```python
from build123d import *

# Parameters (mm, degrees)
F2_R     = 1
F3_SIZE  = 1
F5_DEPTH = 2.88


# Not quite as in the source:
# - a fillet or chamfer that OpenCascade refuses, or shapes differently, is made with other operations: its cross-section is extruded or revolved along the edge and cut away or added


with BuildPart() as f1:
    # F0 (on Front) → F1 (revolve)
    with BuildSketch(Plane.XZ):
        Polygon((-4, 0), (0, 0), (0, 51.056624327), (-2.5, 52.5), (-2.5, 58), (-6.5, 58), (-6.5, 50), (-4, 50), (-4, 46.25), (-3.5, 46), (-4, 45.75), align=None)
    revolve(axis=Axis((0, 0, 18.332445994), (0, 0, 1)))

    # F2
    f2_edges = [f1.edges().sort_by_distance(p)[0] for p in [
        (6.5, 0, 58),
    ]]
    fillet(f2_edges, radius=F2_R)

    # F3
    f3_edges = [f1.edges().sort_by_distance(p)[0] for p in [
        (4, 0, 0),
    ]]
    chamfer(f3_edges, length=F3_SIZE)

    # F4 (on face) → F5 (cut)
    with BuildSketch(Plane.XY.offset(58)):
        Polygon((-1.7320508076, -3), (1.7320508076, -3), (3.4641016151, 0), (1.7320508076, 3), (-1.7320508076, 3), (-3.4641016151, 0), align=None)
    extrude(amount=-F5_DEPTH, mode=Mode.SUBTRACT)

    # F6: chamfer of 1.5 x 2.5980762114 on 1 edges, made by hand


with BuildPart() as f6_tool2:
    # F6_s3 → F6_t4 (revolve)
    with BuildSketch(Plane.XZ):
        Polygon((-5.0980762114, 55.12), (-2.5, 53.62), (-2.5, 55.12), align=None)
    revolve(axis=Axis((0, 0, 55.12), (0, 0, 1)))

    split(bisect_by=Plane(origin=(-2.5980762114, -1.5, 0), x_dir=(0, 0, 1), z_dir=(0.8660254038, 0.5, 0)), keep=Keep.TOP)

    split(bisect_by=Plane(origin=(-2.5980762114, 1.5, 0), x_dir=(0, 0, 1), z_dir=(0.8660254038, -0.5, 0)), keep=Keep.TOP)

    split(bisect_by=Plane.XZ.offset(-3), keep=Keep.TOP)

    split(bisect_by=Plane(origin=(2.5980762114, 1.5, 0), x_dir=(0, 0, 1), z_dir=(-0.8660254038, -0.5, 0)), keep=Keep.TOP)

    split(bisect_by=Plane(origin=(2.5980762114, -1.5, 0), x_dir=(0, 0, 1), z_dir=(-0.8660254038, 0.5, 0)), keep=Keep.TOP)

    split(bisect_by=Plane.XZ.offset(3), keep=Keep.BOTTOM)


with BuildPart() as f1_1:
    add(f1.part)

    # F6_t1: cut F6_tool2
    add(f6_tool2.part, mode=Mode.SUBTRACT)


solid = f1_1.part
```
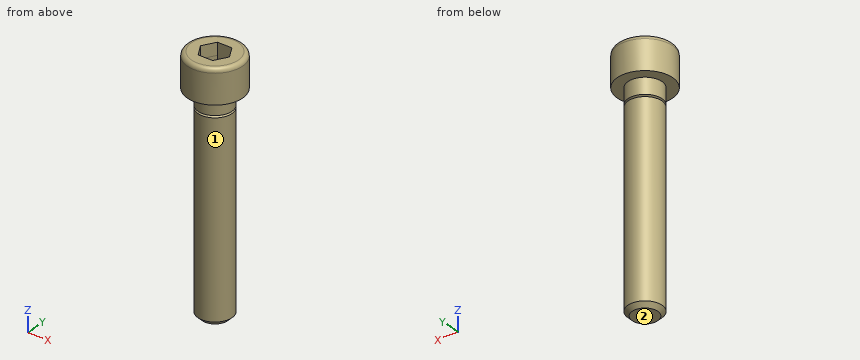
Source: CAD feature listing. Evaluate the final solid. Frame: model axes, mm. Face numbers are marked on the shaded views. A direction names the side the tool comes from. Give positions to 0.01 mm unless a question says otherwise; leave off trailing zeros. Order: outer loops, then holes, each group sorted by start corner. A loop starts at its lowest first (then second) coordinate and runs counter-clockwise, first axis right, second up.
(1) Access query for the marked faces 1 and 2. Directions: +Z, -Z, +X, -X, +Y, -Y. A direction counts if a zero-diameter tool reaches every point of the face in a straight line with its end or side. Return the directions, or none.
(2) Contact query for flat-ended pins moving along their axis: P1, Ø2, axis at x = 3, z = 30.5, coming from the -Y side; P2, Ø5, axis at y = 4.5, z = 43.5, coming from the +X side; P3, Ø5, axis at y = 4.5, z = 37.5, coming from the -X side. Output: stop coordinate, or through.
(3) Material intervals for line 1 along Y through (x, z) = (0, 53.1); line 2 along Z through (x, y) = (-3, -4.25), sorted ascending.
(4) Section query A-A (z = 29). Return the cut outline in (x, y), plus the area to 3 significant figures.
Outcome:
1. face 1: -Z
1. face 2: -Z, +X, -X, +Y, -Y
2. P1: stops at y = -3.46
2. P2: stops at x = 3.46
2. P3: stops at x = -3.46
3. line 1: y = -6.5 to -2.5, 2.5 to 6.5
3. line 2: z = 50 to 58
4. outline: circle Ø8 at (0, 0)
4. area: 50.3 mm2
